from build123d import *

# Parameters (mm, degrees)
F0_W     = 44
F0_H     = 44
F0_W_2   = 39
F0_H_2   = 39
F1_DEPTH = 245
F3_D     = 8.8
F4_W     = 38
F4_H     = 38
F5_DEPTH = 44.001
F7_D     = 8.8


with BuildPart() as f1:
    # F0 (on Top) → F1 (new body)
    with BuildSketch(Plane.XY):
        Rectangle(F0_W, F0_H)
        Rectangle(F0_W_2, F0_H_2, mode=Mode.SUBTRACT)
    extrude(amount=F1_DEPTH)

    # F3 (through all)
    with Locations(Plane(origin=(-22, 0, 0), x_dir=(0, -1, 0), z_dir=(-1, 0, 0))):
        with Locations((0, 195), (-1.2203e-06, 95)):
            Hole(F3_D / 2)

    # F4 (on face) → F5 (cut, through all)
    with BuildSketch(Plane.YZ.offset(22)):
        with Locations((0, 25)):
            Rectangle(F4_W, F4_H)
    extrude(amount=-F5_DEPTH, mode=Mode.SUBTRACT)

    # F7 (through all)
    with Locations(Plane.XZ.offset(22)):
        with Locations((0, 25)):
            Hole(F7_D / 2)


solid = f1.part
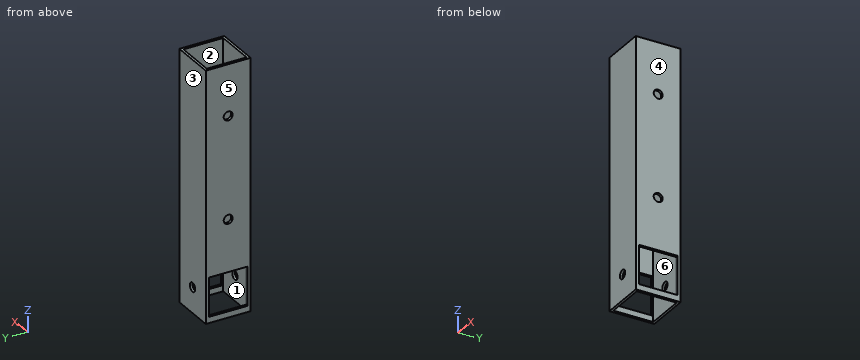
Source: CAD feature listing. Evaluate the final solid. Frame: model axes, mm. Face numbers are marked on the shaded views. A direction names the side the tool comes from. Give positions to 0.01 mm unless a question says otherwise; leave off trailing zeros. Write each loop counter-clockwise with the first axis right and the second up, starting at its lowest first coordinate (ties: lowest second). Pieces come first, ordered by that corner, then holes. Notation, with made-up numbers: (-3.5, 65.25) -> (26.5, 65.25) arc R23 ccw to (26.5, 98.25) -> close; hole circle Ø7 at (-12.5, 69). An arc over 180 degrees is marked (long way). Return JSON: item names as keys, results as strings. Group by question number.
1. Material intervals for line 1 (Z direction, x = -21.3, y = 0); line 2 (Y direction, x = 11, z = 64.5); line 3 (Z direction, x = 0, y = 20.8), sorted ascending. Write a range as from..to.
2. Section B-B, the plane x = 10. Output: boundary loops of the cut face in (y, z), then the cut area to 4 significant figures.
3. Section C-C, the plane z = 195. Output: boundary loops of the cut face in (x, y).
4. Pin query (flat end, axial travel): pin 1 Ø1.2 at (x, y) = (-20, 4) entering from -Z. Return the tip coordinate at first contact, or that it passes through.
5. Access query for the marked faces 5 and 6. Directions: +Z, -Z, +X, -X, +Y, -Y. A direction counts if a zero-diameter tool reaches every point of the face in a straight line with its end or side. Return the directions, or none.
6. Section A-A, the plane y = 0. Count the separate pieces of the cut face and the enclosed holes in it, then the cut area to 3 significant figures.
7. Section D-D, the plane z = 141. Output: boundary loops of the cut face in (x, y), then the cut area to 3 significant figures.
8. Mould query, pull axis Y, two halves, no side actions, for the marked faces 1, 2, 3 and 4. Classes: +Y half, -Y half, draft (parallel to the pull), parting line (faces both ways), or undercut.
Determined:
{
 "1": {"line 1": "z = 0..6, 44..90.6, 99.4..190.6, 199.4..245", "line 2": "y = -22..-19.5, 19.5..22", "line 3": "z = 0..20.6, 29.4..245"},
 "2": {"outline": "(-22, 0) -> (-19.5, 0) -> (-19.5, 245) -> (-22, 245) -> close; (19.5, 0) -> (22, 0) -> (22, 245) -> (19.5, 245) -> close", "area": "1,225 mm2"},
 "3": {"outline": "(-22, -22) -> (22, -22) -> (22, -4.4) -> (19.5, -4.4) -> (19.5, -19.5) -> (-19.5, -19.5) -> (-19.5, -4.4) -> (-22, -4.4) -> close; (-22, 4.4) -> (-19.5, 4.4) -> (-19.5, 19.5) -> (19.5, 19.5) -> (19.5, 4.4) -> (22, 4.4) -> (22, 22) -> (-22, 22) -> close"},
 "4": {"pin 1": "stops at z = 0"},
 "5": {"face 5": "+Z, -Z, -X, +Y, -Y", "face 6": "+Z, -Z"},
 "6": {"separate pieces": "8", "enclosed holes": "0", "area": "947 mm2"},
 "7": {"outline": "(-22, -22) -> (22, -22) -> (22, 22) -> (-22, 22) -> close; hole (-19.5, -19.5) -> (19.5, -19.5) -> (19.5, 19.5) -> (-19.5, 19.5) -> close", "area": "415 mm2"},
 "8": {"face 1": "undercut", "face 2": "undercut", "face 3": "+Y half", "face 4": "draft"}
}
